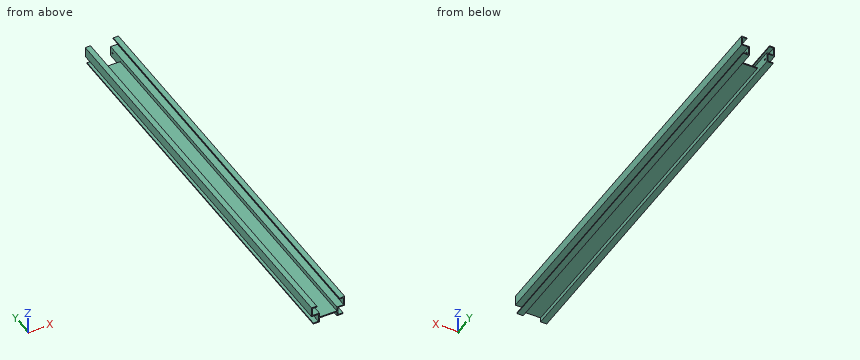
from build123d import *

# Parameters (mm, degrees)
SKETCH1_W                      = 45
SKETCH1_H                      = 2350
BOSS_EXTRUDE1_DEPTH            = 31.5
SKETCH2_W                      = 6
SKETCH2_H                      = 2350
BOSS_EXTRUDE2_DEPTH            = 145
SKETCH3_W                      = 45
SKETCH3_H                      = 2350
BOSS_EXTRUDE3_DEPTH            = 76.5
SKETCH4_W                      = 6
SKETCH4_H                      = 2350
BOSS_EXTRUDE4_DEPTH            = 51
SKETCH5_W                      = 6
SKETCH5_H                      = 2350
BOSS_EXTRUDE5_DEPTH            = 24
SKETCH6_W                      = 15
SKETCH6_H                      = 2350
CUT_EXTRUDE1_DEPTH             = 6
SKETCH7_W                      = 39
SKETCH7_H                      = 2350
CUT_EXTRUDE2_DEPTH             = 45
SKETCH8_W                      = 100
SKETCH8_H                      = 6
CUT_EXTRUDE3_DEPTH             = 100
SKETCH9_W                      = 45
SKETCH9_H                      = 2350
BOSS_EXTRUDE6_DEPTH            = 25.5
SKETCH10_W                     = 39
SKETCH10_H                     = 51
CUT_EXTRUDE4_DEPTH             = 2351
SKETCH11_W                     = 6
SKETCH11_H                     = 2350
BOSS_EXTRUDE7_DEPTH            = 29
SKETCH12_W                     = 45
SKETCH12_H                     = 2350
BOSS_EXTRUDE8_DEPTH            = 25.5
SKETCH13_W                     = 39
SKETCH13_H                     = 51
CUT_EXTRUDE5_DEPTH             = 2351
SKETCH14_W                     = 6
SKETCH14_H                     = 2350
BOSS_EXTRUDE9_DEPTH            = 29
F_10_0_10_DIAMETER_HOLE1_D     = 10
F_10_0_10_DIAMETER_HOLE1_DEPTH = 6
F_10_0_10_DIAMETER_HOLE2_D     = 10
F_10_0_10_DIAMETER_HOLE2_DEPTH = 45


with BuildPart() as part:
    # Sketch1 → Boss-Extrude1 (new body)
    with BuildSketch(Plane(origin=(0, 0, -76.5), x_dir=(-1, 0, 0), z_dir=(0, 0, -1))):
        with Locations((-72.5, 1175)):
            Rectangle(SKETCH1_W, SKETCH1_H)
    extrude(amount=-BOSS_EXTRUDE1_DEPTH)

    # Sketch2 → Boss-Extrude2 (add)
    with BuildSketch(Plane.ZY.offset(-50)):
        with Locations((-73.5, 1175)):
            Rectangle(SKETCH2_W, SKETCH2_H)
    extrude(amount=BOSS_EXTRUDE2_DEPTH)

    # Sketch3 → Boss-Extrude3 (add)
    with BuildSketch(Plane.XY.offset(-70.5)):
        with Locations((-72.5, 1175)):
            Rectangle(SKETCH3_W, SKETCH3_H)
    extrude(amount=BOSS_EXTRUDE3_DEPTH)

    # Sketch4 → Boss-Extrude4 (add)
    with BuildSketch(Plane.XY.offset(-45)):
        with Locations((92, 1175)):
            Rectangle(SKETCH4_W, SKETCH4_H)
    extrude(amount=BOSS_EXTRUDE4_DEPTH)

    # Sketch5 → Boss-Extrude5 (add)
    with BuildSketch(Plane.ZY.offset(-89)):
        with Locations((3, 1175)):
            Rectangle(SKETCH5_W, SKETCH5_H)
    extrude(amount=BOSS_EXTRUDE5_DEPTH)

    # Sketch6 → Cut-Extrude1 (cut)
    with BuildSketch(Plane.XY.offset(6)):
        with Locations((-57.5, 1175)):
            Rectangle(SKETCH6_W, SKETCH6_H)
    extrude(amount=-CUT_EXTRUDE1_DEPTH, mode=Mode.SUBTRACT)

    # Sketch7 → Cut-Extrude2 (cut)
    with BuildSketch(Plane.XY):
        with Locations((-69.5, 1175)):
            Rectangle(SKETCH7_W, SKETCH7_H)
    extrude(amount=-CUT_EXTRUDE2_DEPTH, mode=Mode.SUBTRACT)

    # Sketch8 → Cut-Extrude3 (cut)
    with BuildSketch(Plane(origin=(0, 2350, 0), x_dir=(-1, 0, 0), z_dir=(0, 1, 0))):
        with Locations((0, -73.5)):
            Rectangle(SKETCH8_W, SKETCH8_H)
    extrude(amount=-CUT_EXTRUDE3_DEPTH, mode=Mode.SUBTRACT)

    # Sketch9 → Boss-Extrude6 (add)
    with BuildSketch(Plane(origin=(0, 0, -76.5), x_dir=(-1, 0, 0), z_dir=(0, 0, -1))):
        with Locations((-72.5, 1175)):
            Rectangle(SKETCH9_W, SKETCH9_H)
    extrude(amount=BOSS_EXTRUDE6_DEPTH)

    # Sketch10 → Cut-Extrude4 (cut, through all)
    with BuildSketch(Plane.XZ):
        with Locations((75.5, -76.5)):
            Rectangle(SKETCH10_W, SKETCH10_H)
    extrude(amount=-CUT_EXTRUDE4_DEPTH, mode=Mode.SUBTRACT)

    # Sketch11 → Boss-Extrude7 (add)
    with BuildSketch(Plane(origin=(56, 0, 0), x_dir=(0, 0, -1), z_dir=(1, 0, 0))):
        with Locations((99, 1175)):
            Rectangle(SKETCH11_W, SKETCH11_H)
    extrude(amount=BOSS_EXTRUDE7_DEPTH)

    # Sketch12 → Boss-Extrude8 (add)
    with BuildSketch(Plane(origin=(0, 0, -76.5), x_dir=(-1, 0, 0), z_dir=(0, 0, -1))):
        with Locations((72.5, 1175)):
            Rectangle(SKETCH12_W, SKETCH12_H)
    extrude(amount=BOSS_EXTRUDE8_DEPTH)

    # Sketch13 → Cut-Extrude5 (cut, through all)
    with BuildSketch(Plane(origin=(0, 2350, 0), x_dir=(-1, 0, 0), z_dir=(0, 1, 0))):
        with Locations((75.5, -76.5)):
            Rectangle(SKETCH13_W, SKETCH13_H)
    extrude(amount=-CUT_EXTRUDE5_DEPTH, mode=Mode.SUBTRACT)

    # Sketch14 → Boss-Extrude9 (add)
    with BuildSketch(Plane.ZY.offset(56)):
        with Locations((-99, 1175)):
            Rectangle(SKETCH14_W, SKETCH14_H)
    extrude(amount=BOSS_EXTRUDE9_DEPTH)

    # Ø10.0 (10) Diameter Hole1
    with Locations(Plane.ZY.offset(56)):
        with Locations((-73.5, 2330)):
            Hole(F_10_0_10_DIAMETER_HOLE1_D / 2, depth=F_10_0_10_DIAMETER_HOLE1_DEPTH)

    # Ø10.0 (10) Diameter Hole2
    with Locations(Plane.ZY.offset(-50)):
        with Locations((-73.5, 2330)):
            Hole(F_10_0_10_DIAMETER_HOLE2_D / 2, depth=F_10_0_10_DIAMETER_HOLE2_DEPTH)


solid = part.part
Source: CAD feature listing. Evaluate the final solid. Frame: model axes, mm. Round coordinates to 2 decimals unless told otherwise and drop trailing zeros. Loops run counter-clockwise (first coordinate to the right, second up) from the corner with the lowest first, then second, coordinate; pieces in that order, holes last.
Q1. First-contact query: P1, Ø2, axis at y = 879.5, z = -84.5, coming from the -X side; P2, Ø1.8, axis at y = 1082.5, z = -97.5, coming from the -X side; P3, Ø4, axis at x = -22.5, y = 524.5, coming from the +Z side. Flat tips, straight axial feed; report the tip coordinate or a pass-through.
Q2. Ray query, line 1 (Z direction, x = -80.5, y = 486); line 2 (Z direction, x = -52.8, y = 2330); line 3 (Y direction, x = 52.2, z = -73.5). Return the intervals inside material, ascending.
Q3. Section A-A, the plane y = 313.5. Return loops of the section in (x, z).
Solutions:
1. P1: stops at x = -56
1. P2: stops at x = -85
1. P3: stops at z = -70.5
2. line 1: z = -102 to -96, -51 to -45, 0 to 6
2. line 2: z = -102 to -78.5, -68.5 to -45
2. line 3: y = 0 to 2325, 2335 to 2350
3. outline: (-95, -51) - (-56, -51) - (-56, -96) - (-85, -96) - (-85, -102) - (-50, -102) - (-50, -76.5) - (50, -76.5) - (50, -102) - (85, -102) - (85, -96) - (56, -96) - (56, -51) - (95, -51) - (95, 6) - (65, 6) - (65, 0) - (89, 0) - (89, -45) - (50, -45) - (50, -70.5) - (-50, -70.5) - (-50, -45) - (-89, -45) - (-89, 0) - (-65, 0) - (-65, 6) - (-95, 6) - close
